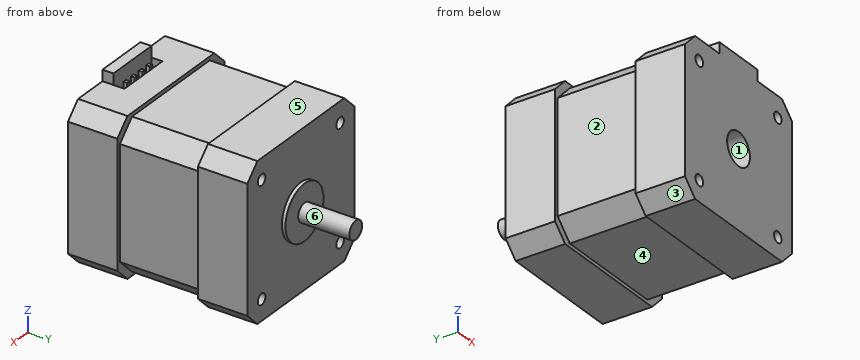
Autodesk Inventor part; units mm, degrees
ref_plane "YZ Plane" through (0, 0, 0) normal (1, 0, 0) x (0, 1, 0)
ref_plane "XZ Plane" through (0, 0, 0) normal (0, 1, 0) x (-1, 0, 0)
ref_plane "XY Plane" through (0, 0, 0) normal (0, 0, 1) x (1, 0, 0)
sketch "Skizze1" plane through (0, 0, 0) normal (0, 1, 0) x (-1, 0, 0)
  line L0 (-21.15, 21.15) -> (21.15, 21.15)
  line L1 (21.15, 21.15) -> (21.15, -21.15)
  line L2 (21.15, -21.15) -> (-21.15, -21.15)
  line L3 (-21.15, -21.15) -> (-21.15, 21.15)
  line L4 (-21.15, 21.15) -> (21.15, -21.15) construction
  line L5 (21.15, 21.15) -> (-21.15, -21.15) construction
  point P0 (0, 0)
  dimension "d0" = 42.3
  dimension "d1" = 42.3
extrude "Extrusion1" add sketch "Skizze1" along normal mid plane 49
sketch "Skizze2" plane through (0, -24.5, 0) normal (0, -1, 0) x (1, 0, 0)
  line L0 (-21.15, 21.15) -> (21.15, 21.15)
  line L1 (-7.5, 21.15) -> (7.5, 21.15)
  line L2 (7.5, 21.15) -> (7.5, 24.15)
  line L3 (7.5, 24.15) -> (-7.5, 24.15)
  line L4 (-7.5, 24.15) -> (-7.5, 21.15)
  line L5 (0, -30.21) -> (0, 33.21)
  point P0 (0, 0)
  dimension "d4" = 15
  dimension "d5" = 3
extrude "Extrusion2" add sketch "Skizze2" against normal blind 3
sketch "Skizze3" plane through (0, -24.5, 0) normal (0, -1, 0) x (1, 0, 0)
  line L0 (-15.5, -15.5) -> (15.5, -15.5)
  line L1 (15.5, -15.5) -> (15.5, 15.5)
  line L2 (15.5, 15.5) -> (-15.5, 15.5)
  line L3 (-15.5, 15.5) -> (-15.5, -15.5)
  line L4 (-15.5, -15.5) -> (15.5, 15.5) construction
  line L5 (15.5, -15.5) -> (-15.5, 15.5) construction
  circle A0 centre (-15.5, 15.5) radius 1.5
  circle A1 centre (15.5, 15.5) radius 1.5
  circle A2 centre (15.5, -15.5) radius 1.5
  circle A3 centre (-15.5, -15.5) radius 1.5
  circle A4 centre (0, 0) radius 4.5
  dimension "d8" = 31
  dimension "d9" = 31
  dimension "d10" = 3
  dimension "d11" = 9
extrude "Extrusion3" cut sketch "Skizze3" along normal through all both and the other way through all contours L3 A3 L0 | L0 A3 L3 | A2 L1 L0 | L0 L1 A2 | A0 L2 L3 | L3 L2 A0 | A1 L2 L1 | L1 L2 A1 | A4
chamfer "Fase1" distance 4 angle 45 4 edges at (21.15, 0, 21.15) (-21.15, 0, 21.15) (21.15, 0, -21.15) (-21.15, 0, -21.15)
sketch "Skizze4" plane through (0, 0, 0) normal (0, 1, 0) x (-1, 0, 0)
  line L0 (20.15, 15.3216) -> (15.3216, 20.15)
  line L1 (-15.3216, 20.15) -> (-20.15, 15.3216)
  line L2 (-20.15, -15.3216) -> (-15.3216, -20.15)
  line L3 (15.3216, -20.15) -> (20.15, -15.3216)
  line L4 (25.5, -25.5) -> (-25.5, -25.5)
  line L5 (-25.5, -25.5) -> (-25.5, 25.5)
  line L6 (-25.5, 25.5) -> (25.5, 25.5)
  line L7 (25.5, 25.5) -> (25.5, -25.5)
  line L8 (25.5, -25.5) -> (-25.5, 25.5) construction
  line L9 (-25.5, -25.5) -> (25.5, 25.5) construction
  line L10 (-21.15, 17.15) -> (-17.15, 21.15)
  line L11 (-17.15, -21.15) -> (-21.15, -17.15)
  line L12 (21.15, -17.15) -> (17.15, -21.15)
  line L13 (17.15, 21.15) -> (21.15, 17.15)
  line L14 (20.15, 15.3216) -> (20.15, -15.3216)
  line L15 (15.3216, -20.15) -> (-15.3216, -20.15)
  line L16 (-20.15, -15.3216) -> (-20.15, 15.3216)
  line L17 (-15.3216, 20.15) -> (15.3216, 20.15)
  line L18 (17.15, 21.15) -> (-17.15, 21.15)
  line L19 (-21.15, 17.15) -> (-21.15, -17.15)
  line L20 (-17.15, -21.15) -> (17.15, -21.15)
  line L21 (21.15, -17.15) -> (21.15, 17.15)
  point P0 (0, 0)
  dimension "d21" = 2
  dimension "d22" = 1
  dimension "d24" = 1
  dimension "d25" = 1
extrude "Extrusion4" cut sketch "Skizze4" along normal mid plane 22 contours L4 L5 L6 L7 | L10 L18 L13 L21 L12 L20 L11 L19
sketch "Skizze6" plane through (-7.5, -21.5, 21.15) normal (0, 0, 1) x (1, 0, 0)
  line L0 (0, 0) -> (15, 0)
  line L1 (15, 0) -> (15, 3)
  line L2 (15, 3) -> (0, 3)
  line L3 (0, 3) -> (0, 0)
  line L4 (15, -3) -> (15, 0)
  line L5 (0, -3) -> (0, 0)
  line L6 (0, 0) -> (15, 0)
  line L7 (2.5, 1) -> (3.5, 1)
  line L8 (3.5, 1) -> (3.5, 2)
  line L9 (3.5, 2) -> (2.5, 2)
  line L10 (2.5, 2) -> (2.5, 1)
  line L11 (2.5, 1) -> (3.5, 2) construction
  line L12 (3.5, 1) -> (2.5, 2) construction
  line L13 (5.5, 1) -> (6.5, 1)
  line L14 (6.5, 1) -> (6.5, 2)
  line L15 (6.5, 2) -> (5.5, 2)
  line L16 (5.5, 2) -> (5.5, 1)
  line L17 (5.5, 1) -> (6.5, 2) construction
  line L18 (6.5, 1) -> (5.5, 2) construction
  line L19 (8.5, 1) -> (9.5, 1)
  line L20 (9.5, 1) -> (9.5, 2)
  line L21 (9.5, 2) -> (8.5, 2)
  line L22 (8.5, 2) -> (8.5, 1)
  line L23 (8.5, 1) -> (9.5, 2) construction
  line L24 (9.5, 1) -> (8.5, 2) construction
  line L25 (11.5, 1) -> (12.5, 1)
  line L26 (12.5, 1) -> (12.5, 2)
  line L27 (12.5, 2) -> (11.5, 2)
  line L28 (11.5, 2) -> (11.5, 1)
  line L29 (11.5, 1) -> (12.5, 2) construction
  line L30 (12.5, 1) -> (11.5, 2) construction
  line L31 (7.5, -12.8) -> (7.5, 55.8)
  point P0 (7.5, 21.5)
  point P1 (3, 1.5)
  point P2 (6, 1.5)
  point P3 (9, 1.5)
  point P4 (12, 1.5)
  point P5 (12, 1.5)
  point P6 (15, 1.5)
  dimension "d29" = 3
  dimension "d30" = 3
  dimension "d31" = 3
  dimension "d32" = 1
  dimension "d33" = 1
extrude "Extrusion6" cut sketch "Skizze6" against normal blind 5
sketch "Skizze7" plane through (0, 0, 0) normal (1, 0, 0) x (0, 1, 0)
  line L0 (39.5, 0) -> (39.5, 2.5)
  line L1 (39.5, 2.5) -> (25.5, 2.5)
  line L2 (25.5, 2.5) -> (25.5, 7.5)
  line L3 (25.5, 7.5) -> (24.5, 7.5)
  line L4 (24.5, -17.15) -> (24.5, 17.15)
  line L5 (24.5, 0) -> (39.5, 0)
  line L6 (24.5, 0) -> (24.5, 7.5)
  line L7 (38.5419, 0) -> (33.7383, 0)
  point P0 (0, 0)
  dimension "d37" = 5
  dimension "d38" = 1
  dimension "d39" = 15
  dimension "d40" = 15
revolve "Umdrehung1" add sketch "Skizze7" angle 360 about axis through (0, 24.5, 0) along (0, 1, 0)
equation "\"d24\" = d22"
equation "\"d25\" = d22"
equation "\"d33\" = d32"
properties part number "Nema17drylin"
Source: CAD feature listing. Evaluate the final solid. Frame: model axes, mm. Face numbers are marked on the shaded views. A direction names the side the tool comes from. Round coordinates to 2 decimals unless told otherwise and drop trailing zeros. Loops run counter-clockwise (first coordinate to the right, second up) from the corner with the lowest first, then second, coordinate; pieces in that order, holes last. Notation, with made-up numbers: M -7,55.25 L -3,55.25 A16 cw -3,85.25 Z; hole C -39.75,61 d8. An arc over 180 degrees is marked long. Return JSON: item names as keys, results as strings. Group by question number.
1. Section query C-C on x = 6. Output: boundary loops of the cut face in (y, z).
2. Section query D-D on x = -11.5. Output: boundary loops of the cut face in (y, z), and give its area (3 significant figures).
3. Mould query, pull axis Z, two halves, no side actions, for the marked faces 1, 2 and 3. Classes: released by +Z, released by -Z, zero draft, split by the parting line, or undercut.
4. Pin query (flat end, axial travel): pin 1 (0.5 mm diameter, centred on x = 1.5, z = 18.5, fed in from +Y); pin 2 (11 mm diameter, centred on x = -7, y = -1, fed in from +Z); pin 3 (1.1 mm diameter, centred on y = -20, z = 18, fed in from -X). Return the tip coordinate at first contact, or that it passes through.
5. Section query B-B on x = 0. Output: boundary loops of the cut face in (y, z).
6. Section query A-A on y = 8.5. Output: boundary loops of the cut face in (x, z), and give its area (3 significant figures).
7. Material intervals for line 1 along Z through (x, y) = (0, 13); line 2 along X through (y, z) = (-4, -15.5), sorted ascending. Write a range as from..to.
8. Reachability of the marked faces 4, 5 and 6 from +Z, -Z, +X, -X, +Y, -Y: full face, straight path, thin tool, end or side. Return the list, or none.
Checks:
{
 "1": {"outline": "M -24.5,-21.15 L -11,-21.15 L -11,-20.15 L 11,-20.15 L 11,-21.15 L 24.5,-21.15 L 24.5,-4.5 L 25.5,-4.5 L 25.5,4.5 L 24.5,4.5 L 24.5,21.15 L 11,21.15 L 11,20.15 L -11,20.15 L -11,21.15 L -18.5,21.15 L -18.5,16.15 L -21.5,16.15 L -21.5,24.15 L -24.5,24.15 Z"},
 "2": {"outline": "M -24.5,-21.15 L -11,-21.15 L -11,-20.15 L 11,-20.15 L 11,-21.15 L 24.5,-21.15 L 24.5,21.15 L 11,21.15 L 11,20.15 L -11,20.15 L -11,21.15 L -24.5,21.15 Z", "area": "2,030 mm²"},
 "3": {"face 1": "undercut", "face 2": "zero draft", "face 3": "released by -Z"},
 "4": {"pin 1": "stops at y = 24.5", "pin 2": "stops at z = 20.15", "pin 3": "stops at x = -20.85"},
 "5": {"outline": "M -24.5,-21.15 L -11,-21.15 L -11,-20.15 L 11,-20.15 L 11,-21.15 L 24.5,-21.15 L 24.5,-7.5 L 25.5,-7.5 L 25.5,-2.5 L 39.5,-2.5 L 39.5,2.5 L 25.5,2.5 L 25.5,7.5 L 24.5,7.5 L 24.5,21.15 L 11,21.15 L 11,20.15 L -11,20.15 L -11,21.15 L -18.5,21.15 L -18.5,16.15 L -21.5,16.15 L -21.5,24.15 L -24.5,24.15 L -24.5,4.5 L 24.5,4.5 L 24.5,-4.5 L -24.5,-4.5 Z"},
 "6": {"outline": "M -20.15,-15.32 L -15.32,-20.15 L 15.32,-20.15 L 20.15,-15.32 L 20.15,15.32 L 15.32,20.15 L -15.32,20.15 L -20.15,15.32 Z; hole C -15.5,-15.5 d3; hole C -15.5,15.5 d3; hole C 0,0 d9; hole C 15.5,-15.5 d3; hole C 15.5,15.5 d3", "area": "1,490 mm²"},
 "7": {"line 1": "z = -21.15..-4.5, 4.5..21.15", "line 2": "x = -19.97..-17, -14..14, 17..19.97"},
 "8": {"face 4": "-Z, +X, -X", "face 5": "+Z, +X, -X, +Y", "face 6": "+Y"}
}
